Verification items for the finished model (mm, model axes). A direction names the side the tool comes from. Round coordinates to 2 decimals unless told otherwise and drop trailing zeros. Loops run counter-clockwise (first coordinate to the right, second up) from the corner with the lowest first, then second, coordinate; pieces in that order, holes last. Notation, with made-up numbers: (26.25, 36.25) -> (79.25, 36.25) arc R33 ccw to (79.25, 69.25) -> close; hole circle Ø2 at (34.5, 54.5). An arc over 180 degrees is marked (long way). Use a Markdown table: item, result. Add a question column.
```python
from build123d import *

# Parameters (mm, degrees)
F1_DEPTH = 25
F3_DEPTH = 5.08
F5_DEPTH = 5.08
F6_R     = 9.328151
F7_DEPTH = 30.001


with BuildPart() as f1:
    # F0 (on Front) → F1 (new body, symmetric)
    with BuildSketch(Plane.XZ):
        Polygon((-15, 0), (0, 0), (15, 0), (15, 6.35), (15, 12.947081), (9.92, 12.947081), (9.92, 6.35), (0, 6.35), (-9.92, 6.35), (-9.92, 12.947081), (-15, 12.947081), (-15, 6.35), align=None)
    extrude(amount=F1_DEPTH, both=True)

    # F2 (on face) → F3 (join)
    with BuildSketch(Plane.YZ.offset(15)):
        Polygon((25, 12.947081), (25, 40), (0, 40), (-25, 12.947081), align=None)
    extrude(amount=-F3_DEPTH)

    # F4 (on face) → F5 (join)
    with BuildSketch(Plane(origin=(-15, 0, 0), x_dir=(0, -1, 0), z_dir=(-1, 0, 0))):
        Polygon((-25, 40.16066), (-25, 12.947081), (0, 12.947081), (25, 12.947081), (0, 40.16066), align=None)
    extrude(amount=-F5_DEPTH)

    # F6 (on face) → F7 (cut, through all)
    with BuildSketch(Plane(origin=(-15, 0, 0), x_dir=(0, -1, 0), z_dir=(-1, 0, 0))):
        with Locations((-12.660467, 23.76432)):
            Circle(F6_R)
    extrude(amount=-F7_DEPTH, mode=Mode.SUBTRACT)


solid = f1.part
```
1) Sectioned sample at A-A on z = 12. Enter the section's corners in (x, y), then the cut area to 3 significant figures.
2) Go/stop test with flat-tipped pins: pin 1 (2.5 mm diameter, centred on x = 11.5, y = 9.5, fed in from +Z); pin 2 (4 mm diameter, centred on x = -7, y = 6, fed in from +Z). Record where each tip stops, or that it passes through.
3) Sectioned sample at D-D on x = 12.25. Enter the section's corners in (y, z).
4) Thickness scan on line 1 (X direction, y = -20.5, z = 7); line 2 (Z direction, x = -3.75, y = 10.5); line 3 (Y direction, x = 12.5, z = 18). Record the ranges inside material, lowest first.
5) Sectioned sample at C-C on y = 10.5. Enter the section's corners in (x, z), then the cut area to 3 significant figures.
6) Release check for a two-part mould opening along X. For faces 4 (the face through (0, 0, 6.35)), 5 (the face through (12, 13, 40)), 6 (the face through (-15, 0, 16)) record: released by +X, released by -X, zero draft, split by the parting line, or undercut.
7) Sectioned sample at B-B on z = 16.5. Enter the section's corners in (x, y).
8) Access from +Z, -Z, +X, -X, +Y, -Y to the whole of each face (thin tool, end or side, straight path). Record for faces 1 (the face through (12.5, -12.33, 26.66)), 2 (the face through (9.92, 0, 20)), 3 (the face through (-12.496, -12.675, 26.363)).
Geometry results:
| question | item | result |
|---|---|---|
| 1 | outline | (-15, -25) -> (-9.92, -25) -> (-9.92, 25) -> (-15, 25) -> close; (9.92, -25) -> (15, -25) -> (15, 25) -> (9.92, 25) -> close |
| 1 | area | 508 mm^2 |
| 2 | pin 1 | z = 40 |
| 2 | pin 2 | z = 6.35 |
| 3 | outline | (-25, 0) -> (25, 0) -> (25, 40) -> (0, 40) -> (-25, 12.95) -> close; hole circle Ø18.66 at (12.66, 23.76) |
| 4 | line 1 | -15 to -9.92, 9.92 to 15 |
| 4 | line 2 | 0 to 6.35 |
| 4 | line 3 | -20.33 to 5.33, 19.99 to 25 |
| 5 | outline | (-15, 0) -> (15, 0) -> (15, 14.69) -> (9.92, 14.69) -> (9.92, 6.35) -> (-9.92, 6.35) -> (-9.92, 14.69) -> (-15, 14.69) -> close; (-15, 32.84) -> (-9.92, 32.84) -> (-9.92, 40.16) -> (-15, 40.16) -> close; (9.92, 32.84) -> (15, 32.84) -> (15, 40) -> (9.92, 40) -> close |
| 5 | area | 349 mm^2 |
| 6 | face 4 | undercut |
| 6 | face 5 | zero draft |
| 6 | face 6 | released by -X |
| 7 | outline | (-15, -21.74) -> (-9.92, -21.74) -> (-9.92, 6.81) -> (-15, 6.81) -> close; (-15, 18.51) -> (-9.92, 18.51) -> (-9.92, 25) -> (-15, 25) -> close; (9.92, -21.72) -> (15, -21.72) -> (15, 6.81) -> (9.92, 6.81) -> close; (9.92, 18.51) -> (15, 18.51) -> (15, 25) -> (9.92, 25) -> close |
| 8 | face 1 | +Z, +X, -Y |
| 8 | face 2 | +Z, +Y, -Y |
| 8 | face 3 | +Z, +X, -X, -Y |
